Check sheet for the modelled part. Datum: model origin and axes. Units: mm. A direction names the side the tool comes from. Round coordinates to 2 decimals unless told otherwise and drop trailing zeros. Order: outer loops, then holes, each group sorted by start corner. A loop starts at its lowest first (then second) coordinate and runs counter-clockwise, first axis right, second up. Notation, with made-up numbers: (25.5, 80.5) -> (31.5, 80.5) arc R36 ccw to (31.5, 115.5) -> close; hole circle Ø6 at (27.5, 60). An arc over 180 degrees is marked (long way). Answer in a Markdown table with one row per item.
```python
from build123d import *

# Parameters (mm, degrees)
SKETCH_1_W                       = 85
SKETCH_1_H                       = 15
SM_BASE_FLANGE_1_DEPTH           = 1
SM_EDGE_FLANGE_1_STRIP_W         = 6
SM_EDGE_FLANGE_1_STRIP_H         = 1
SM_EDGE_FLANGE_1_STRIP_CUT_DEPTH = 85
SM_EDGE_FLANGE_1_DEPTH           = 85
SKETCH_9_R                       = 2.1
CUT_EXTRUDE_1_DEPTH              = 10
HOLE_WIZARD_M31_D                = 3.4
HOLE_WIZARD_M31_DEPTH            = 18.5
HOLE_WIZARD_M31_TIP              = 1.021463052


# Sheet-metal steps are written as plain solids
with BuildPart() as part:
    # Sketch 1 → Базовая кромка1 (new body)
    with BuildSketch(Plane.XY):
        Rectangle(SKETCH_1_W, SKETCH_1_H)
    extrude(amount=-SM_BASE_FLANGE_1_DEPTH)

    # Ребро-кромка1 strip (across the edge) → Ребро-кромка1 strip cut (cut)
    with BuildSketch(Plane(origin=(42.5, 7.5, 0), x_dir=(0, -1, 0), z_dir=(-1, 0, 0))):
        with Locations((-1, -0.5)):
            Rectangle(SM_EDGE_FLANGE_1_STRIP_W, SM_EDGE_FLANGE_1_STRIP_H)
    extrude(amount=SM_EDGE_FLANGE_1_STRIP_CUT_DEPTH, mode=Mode.SUBTRACT)

    # Ребро-кромка1 section (across the edge) → Ребро-кромка1 (add)
    with BuildSketch(Plane(origin=(42.5, 7.5, 0), x_dir=(0, -1, 0), z_dir=(-1, 0, 0))):
        with BuildLine():
            Line((0, 1), (0, 13))
            Line((0, 13), (1, 13))
            Line((1, 13), (1, 1))
            ThreePointArc((1, 1), (1.292893219, 0.292893219), (2, 0))
            Line((2, 0), (2, -1))
            ThreePointArc((2, -1), (0.585786438, -0.414213562), (0, 1))
        make_face()
    extrude(amount=SM_EDGE_FLANGE_1_DEPTH)

    # Эскиз9 → Вырез-Вытянуть1 (cut)
    with BuildSketch(Plane.XY):
        with Locations((-27.5, 0)):
            Circle(SKETCH_9_R)
        with Locations((27.5, 0)):
            Circle(SKETCH_9_R)
    extrude(amount=-CUT_EXTRUDE_1_DEPTH, mode=Mode.SUBTRACT)

    # Отверстие с зазором M31
    with Locations(Plane(origin=(0, 6.5, 0), x_dir=(-1, 0, 0), z_dir=(0, -1, 0))):
        with Locations((-35, -7), (35, -7)):
            Hole(HOLE_WIZARD_M31_D / 2, depth=HOLE_WIZARD_M31_DEPTH)
            with Locations((0, 0, -(HOLE_WIZARD_M31_DEPTH + HOLE_WIZARD_M31_TIP / 2))):  # 118° drill point
                Cone(0, HOLE_WIZARD_M31_D / 2, HOLE_WIZARD_M31_TIP, mode=Mode.SUBTRACT)


solid = part.part
```
(1) Tool access check on faces 1 (the cylindrical face through (35.8, 7, 8.5)), 2 (the flat face through (-1, -1, 0)). Record the directions out of +Z, -Z, +X, -X, +Y, -Y that give a thin tool (end or side, any length) a straight path to the whole face; none if there is none.
Solutions:
| item | result |
|---|---|
| face 1 | +Y, -Y |
| face 2 | +Z, +X, -X, -Y |
(2) Scan lines: probe 1 along X at (y, z) = (7.2, 7); probe 2 along Y at (x, z) = (25.5, 4.75); probe 3 along Z at (x, y) = (-31.5, 4.75). Record each from-to range of solid material in increasing order. Write a range as from..to.
Solutions:
| item | result |
|---|---|
| probe 1 | -42.5..-36.7, -33.3..33.3, 36.7..42.5 |
| probe 2 | 6.5..7.5 |
| probe 3 | -1..0 |
(3) Section check D-D on y = -4.75. Record the boundary of the cut face in (x, z).
Solutions:
| item | result |
|---|---|
| outline | (-42.5, -1) -> (42.5, -1) -> (42.5, 0) -> (-42.5, 0) -> close |
(4) Section check B-B on x = -35. Record the boundary of the cut face in (y, z).
Solutions:
| item | result |
|---|---|
| outline | (-7.5, -1) -> (5.5, -1) arc R2 ccw to (7.5, 1) -> (7.5, 5.3) -> (6.5, 5.3) -> (6.5, 1) arc R1 cw to (5.5, 0) -> (-7.5, 0) -> close; (6.5, 8.7) -> (7.5, 8.7) -> (7.5, 13) -> (6.5, 13) -> close |
(5) Draft check along X on faces 3 (the flat face through (42.5, 3.3, -0.2)), 4 (the flat face through (-1, -1, -1)), 5 (the cylindrical face through (-34.2, 7, 8.5)), 6 (the flat face through (-42.5, 3.3, -0.2)). Enter one of: pulls with the +X half, pulls with the -X half, needs draft (parallel to the pull), parting line crosses it, or undercut.
Solutions:
| item | result |
|---|---|
| face 3 | pulls with the +X half |
| face 4 | needs draft |
| face 5 | undercut |
| face 6 | pulls with the -X half |
(6) Depth check by flat-ended pin: pin 1 Ø4 at (x, y) = (27.5, 0) entering from +Z; pin 2 Ø6.5 at (x, y) = (-27.5, 0) entering from +Z; pin 3 Ø4 at (x, z) = (-35, 7) entering from -Y. Enter the tip coordinate at first touch or a pass-through.
Solutions:
| item | result |
|---|---|
| pin 1 | through |
| pin 2 | z = 0 |
| pin 3 | y = 6.5 |
(7) Section check C-C on x = 19. Record the boundary of the cut face in (y, z).
Solutions:
| item | result |
|---|---|
| outline | (-7.5, -1) -> (5.5, -1) arc R2 ccw to (7.5, 1) -> (7.5, 13) -> (6.5, 13) -> (6.5, 1) arc R1 cw to (5.5, 0) -> (-7.5, 0) -> close |
(8) Section check A-A on z = 7. Record the boundary of the cut face in (x, y), plus the area to 3 significant figures.
Solutions:
| item | result |
|---|---|
| outline | (-42.5, 6.5) -> (-36.7, 6.5) -> (-36.7, 7.5) -> (-42.5, 7.5) -> close; (-33.3, 6.5) -> (33.3, 6.5) -> (33.3, 7.5) -> (-33.3, 7.5) -> close; (36.7, 6.5) -> (42.5, 6.5) -> (42.5, 7.5) -> (36.7, 7.5) -> close |
| area | 78.2 mm^2 |
